Autodesk Inventor part; units mm, degrees
ref_plane "YZ Plane" through (0, 0, 0) normal (1, 0, 0) x (0, 1, 0)
ref_plane "XZ Plane" through (0, 0, 0) normal (0, 1, 0) x (-1, 0, 0)
ref_plane "XY Plane" through (0, 0, 0) normal (0, 0, 1) x (1, 0, 0)
sketch "Sketch1" plane through (0, 0, 0) normal (0, 0, 1) x (1, 0, 0)
  line L0 (-6.5, 53.5) -> (0, 53.5)
  line L1 (-20, 57.5) -> (-10.5, 57.5)
  line L2 (-6.5, 53.5) -> (-10.5, 53.5) construction
  line L3 (-10.5, 53.5) -> (-10.5, 57.5) construction
  line L4 (-6.5, 53.5) -> (-10.5, 57.5)
  line L5 (-20, 57.5) -> (-20, 47.5)
  line L6 (0, 53.5) -> (0, 0) construction
  line L7 (0, 0) -> (-10, 0)
  line L8 (-20, 47.5) -> (-10, 37.5)
  line L9 (-20, 47.5) -> (-5.8579, 47.5) construction
  line L10 (-10, 0) -> (-10, 37.5)
  line L11 (6.5, 53.5) -> (0, 53.5)
  line L12 (20, 57.5) -> (10.5, 57.5)
  line L13 (6.5, 53.5) -> (10.5, 53.5) construction
  line L14 (10.5, 53.5) -> (10.5, 57.5) construction
  line L15 (6.5, 53.5) -> (10.5, 57.5)
  line L16 (20, 57.5) -> (20, 47.5)
  line L17 (0, 0) -> (10, 0)
  line L18 (20, 47.5) -> (10, 37.5)
  line L19 (20, 47.5) -> (5.8579, 47.5) construction
  line L20 (10, 0) -> (10, 37.5)
  dimension "d0" = 6.5
  dimension "d1" = 9.5
  dimension "d2" = 4
  dimension "d3" = 4
  dimension "d5" = 10
  dimension "d6" = 53.5
  dimension "d7" = 10
  dimension "d8" = 45
extrude "Extrusion1" add sketch "Sketch1" along normal blind 10
sketch "Sketch2" plane through (-10, 0, 0) normal (-1, 0, 0) x (0, 0, 1)
  line L0 (0, 0) -> (10, 0) construction
  line L1 (5, 0) -> (5, 15) construction
  line L2 (5, 0) -> (-20, 0)
  line L3 (5, 0) -> (30, 0)
  line L4 (-20, 0) -> (-20, 5)
  line L5 (-20, 5) -> (5, 15)
  line L6 (30, 0) -> (30, 5)
  line L7 (30, 5) -> (5, 15)
  dimension "d11" = 15
  dimension "d12" = 25
  dimension "d15" = 5
extrude "Extrusion2" add sketch "Sketch2" against normal up to surface (20 mm away)
sketch "Sketch3" plane through (-6.5, 53.5, 0) normal (0, 1, 0) x (1, 0, 0)
  line L0 (-3.5, -30) -> (16.5, -30)
  line L1 (6.5, -30) -> (6.5, 20) construction
  line L2 (-3.5, 20) -> (16.5, 20)
  line L3 (-13.5, 0) -> (-13.5, -10) construction
  line L4 (-13.5, -5) -> (26.5, -5) construction
  line L5 (26.5, 0) -> (26.5, -10) construction
  line L6 (-3.5, 20) -> (-3.5, -30) construction
  line L7 (-3.5, -25) -> (16.5, -25) construction
  line L8 (16.5, -30) -> (16.5, -10) construction
  circle A0 centre (6.5, -25) radius 1.75
  circle A1 centre (6.5, 15) radius 1.75
  point P0 (6.5, 0)
  dimension "d16" = 5
  dimension "d17" = 3.5
extrude "Extrusion3" cut sketch "Sketch3" against normal through all
sketch "Sketch4" plane through (-10, 0, 30) normal (0, -1, 0) x (1, 0, 0)
  line L0 (20, -50) -> (20, 0) construction
  line L1 (20, -25) -> (0, -25) construction
  line L2 (0, -50) -> (0, 0) construction
  circle A0 centre (10, -5) radius 1.75
  circle A1 centre (10, -5) radius 3
  circle A2 centre (10, -45) radius 3
  circle A3 centre (10, -45) radius 1.75
  point P0 (10, -30)
  dimension "d20" = 6
extrude "Extrusion4" add sketch "Sketch4" against normal blind 9
properties part number "aux_axis_support"
CAD build for the part. Positions are in the model's coordinates, mm. A direction names the side the tool comes from. Coordinates: 2 decimals unless noted, no trailing zeros. Loops run counter-clockwise (first coordinate to the right, second up) from the corner with the lowest first, then second, coordinate; pieces in that order, holes last. Notation, with made-up numbers: (-23, 84) - (21, 84) arc R26 cw to (21, 101) - close; hole circle Ø6 at (-12.5, -23). An arc over 180 degrees is marked (long way). Use one line per item in the form item = value. Start each with the question number.
1) Flat gauge pins, fed straight in: pin 1 (1.5 mm diameter, centred on x = -1, z = 14, fed in from +Y); pin 2 (5.5 mm diameter, centred on x = 0, z = -15, fed in from -Y); pin 3 (12 mm diameter, centred on x = 10.5, y = 24, fed in from +Z); pin 4 (8 mm diameter, centred on x = -1, z = 3, fed in from +Y). Where does each tip first touch, or does it go through?
2) Band-saw the part on A-A (x = 0). Give the cut face in (y, z), and give its area (3 significant figures).
3) Band-saw the part on B-B (z = 25). Give the cut face in (x, y), and give its area (4 significant figures).
4) Two-plate mould, pull along X, no slides. Class faces 1 (the face through (-15.1, 42.6, 4.9)), 2 (the face through (15.1, 42.6, 4.9)), 3 (the face through (0, 53.5, 5)), 4 (the face through (8, 55, 5)): +X half, -X half, draft (parallel to the pull), parting line (faces both ways), or undercut.
5) Tool access for faces 5 (the face through (-10, 12, 7)), 6 (the face through (0, 36, 0)), 7 (the face through (-8, 55, 5)), 8 (the face through (0, 36, 10)): list every direction of +Z, -Z, +X, -X, +Y, -Y with a clear straight run to the whole face (end or side of a thin tool).
6) Band-saw the part on C-C (y = 28.5). Give the cut face in (x, z), and give its area (3 significant figures).
7) Drill centre lines: L1, parallel to Z at x = 0, y = 4.25; L2, parallel to Z at x = 0, y = 6.5; L3, parallel to X at y = 4, z = -15. Where is each one in solid material? Low to high. Write a range as from..to.
8) Band-saw the part on D-D (z = 5.5). Give the cut face in (x, y).
Check values:
q1.pin_1 = 11.7
q1.pin_2 = 0
q1.pin_3 = 10
q1.pin_4 = 53.5
q2.outline = (0, -20) - (5, -20) - (5.8, -18) - (9, -18) - (9, -16.75) - (0, -16.75) - close; (0, -13.25) - (9, -13.25) - (9, -12) - (8.2, -12) - (13, 0) - (53.5, 0) - (53.5, 10) - (13, 10) - (8.2, 22) - (9, 22) - (9, 23.25) - (0, 23.25) - close; (0, 26.75) - (9, 26.75) - (9, 28) - (5.8, 28) - (5, 30) - (0, 30) - close
q2.area = 856 mm2
q3.outline = (-10, 0) - (-1.75, 0) - (-1.75, 9) - (-3, 9) - (-3, 7) - (-10, 7) - close; (1.75, 0) - (10, 0) - (10, 7) - (3, 7) - (3, 9) - (1.75, 9) - close
q3.area = 120.5 mm2
q4.face_1 = -X half
q4.face_2 = +X half
q4.face_3 = undercut
q4.face_4 = undercut
q5.face_5 = +Z, -Z, -X, -Y
q5.face_6 = -Z, +X, -X, +Y
q5.face_7 = +Z, -Z, +Y
q5.face_8 = +Z, +X, -X, +Y
q6.outline = (-10, 0) - (10, 0) - (10, 10) - (-10, 10) - close
q6.area = 200 mm2
q7.L1 = -20..-16.75, -13.25..23.25, 26.75..30
q7.L2 = -18..-16.75, -13.25..23.25, 26.75..28
q7.L3 = -10..-1.75, 1.75..10
q8.outline = (-20, 47.5) - (-10, 37.5) - (-10, 0) - (10, 0) - (10, 37.5) - (20, 47.5) - (20, 57.5) - (10.5, 57.5) - (6.5, 53.5) - (-6.5, 53.5) - (-10.5, 57.5) - (-20, 57.5) - close
